Input: part model. Units: mm. Frame: model coordinates. Face numbers are marked on the shaded views. A direction names the side the tool comes from. Coordinates: 2 decimals unless noted, no trailing zeros. Write each loop counter-clockwise with the first axis right and the second up, starting at its lowest first coordinate (ties: lowest second). Pieces come first, ordered by that corner, then holes. Notation, with made-up numbers: (70, 75) - (118, 75) arc R29 ccw to (118, 107) - close; hole circle Ø11 at (-34, 15). An arc over 180 degrees is marked (long way). One line per question, with ' | ' between items. Start each with the question number.
1) First-contact query: P1, Ø3, axis at x = 81, z = -27.5, coming from the -Y side; P2, Ø9.5, axis at x = -136.5, z = -240, coming from the +Y side; P3, Ø15, axis at x = -132.5, z = -236, coming from the -Y side. Flat tips, straight axial feed; report the tip coordinate or a pass-through.
2) Draft query along Z for the marked faces 4, 5, 6 and 7. Return one class per face: released by +Z, released by -Z, zero draft, split by the parting line, or undercut.
3) Line query: line 1 (Y direction, x = 48.5, z = -10); line 2 (X direction, y = -253, z = 18); line 3 (X direction, y = 6.5, z = 45). Output: solid intervals per line, ascending.
4) Section query B-B on x = 0. Return loops of the section in (y, z), and give its area (3 significant figures).
5) Section query A-A on z = 0. Return loops of the section in (x, y).
6) Section query C-C on y = -152.5. Return loops of the section in (x, z).
7) Reachability of the marked faces 1, 2 and 3 from +Z, -Z, +X, -X, +Y, -Y: full face, straight path, thin tool, end or side. Return the list, or none.
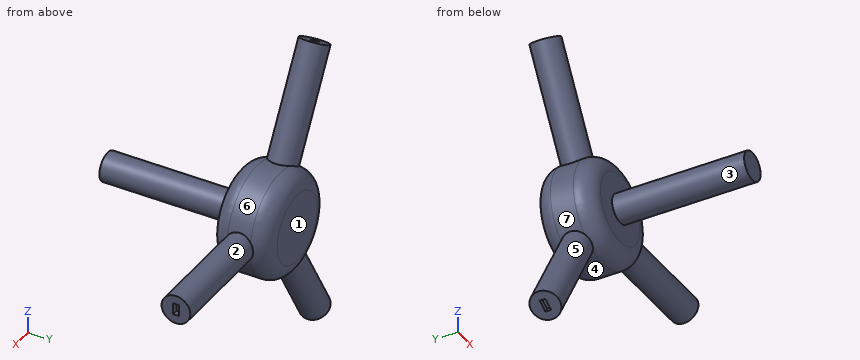
```python
from build123d import *

# Parameters (mm, degrees)
SKETCH_1_W               = 25
SKETCH_1_H               = 230
SKETCH_5_R               = 25
EXTRUDE_1_DEPTH          = 280
PATTERN_CIRCULAR_1_COUNT = 3
SKETCH_7_W               = 20
SKETCH_7_H               = 10
CUT_EXTRUDE_2_DEPTH      = 10
PATTERN_CIRCULAR_2_COUNT = 3


with BuildPart() as part:
    # 草图1 → 旋转1 (revolve)
    with BuildSketch(Plane.XY, mode=Mode.PRIVATE) as revolve_1_sk:
        with BuildLine():
            Line((90, -20), (90, 20))
            ThreePointArc((90, 20), (81.213203436, 41.213203436), (60, 50))
            Line((60, 50), (0, 50))
            Line((0, 50), (0, -50))
            Line((0, -50), (60, -50))
            ThreePointArc((60, -50), (81.213203436, -41.213203436), (90, -20))
        make_face()
        with Locations((12.5, -165)):
            Rectangle(SKETCH_1_W, SKETCH_1_H)
    revolve(revolve_1_sk.sketch.rotate(Axis((0, 124, 0), (0, -1, 0)), 90), axis=Axis((0, 124, 0), (0, -1, 0)))

    # 草图5 → 凸台-拉伸1 (add)
    with BuildSketch(Plane(origin=(0, 0, 0), x_dir=(0, 0, -1), z_dir=(1, 0, 0))):
        with Locations(Location((0, 0, 0), (0, 0, 126.869897646))):
            Circle(SKETCH_5_R)
    extrude_1 = extrude(amount=EXTRUDE_1_DEPTH)

    # 阵列(圆周)1: 凸台-拉伸1 ×3 about axis
    pattern_circular_1_axis = Axis((0, 0, 0), (0, 1, 0))
    for i in range(1, PATTERN_CIRCULAR_1_COUNT):
        add(extrude_1.rotate(pattern_circular_1_axis, i * 360 / PATTERN_CIRCULAR_1_COUNT))

    # 草图7 → 切除-拉伸2 (cut)
    with BuildSketch(Plane(origin=(280, 0, 0), x_dir=(0, 0, -1), z_dir=(1, 0, 0))):
        Rectangle(SKETCH_7_W, SKETCH_7_H)
    cut_extrude_2 = extrude(amount=-CUT_EXTRUDE_2_DEPTH, mode=Mode.SUBTRACT)

    # 阵列(圆周)2: 切除-拉伸2 ×3 about axis
    pattern_circular_2_axis = Axis((0, 0, 0), (0, 1, 0))
    for i in range(1, PATTERN_CIRCULAR_2_COUNT):
        add(cut_extrude_2.rotate(pattern_circular_2_axis, i * 360 / PATTERN_CIRCULAR_2_COUNT), mode=Mode.SUBTRACT)


solid = part.part
```
Answer key:
1) P1: y = -37.95 | P2: y = 25 | P3: y = -25
2) face 4: released by -Z | face 5: undercut | face 6: released by +Z | face 7: undercut
3) line 1: -50 to 50 | line 2: -17.35 to 17.35 | line 3: -77.94 to 77.94
4) outline: (-280, -25) - (-50, -25) - (-50, -60) arc R30 ccw to (-20, -90) - (20, -90) arc R30 ccw to (50, -60) - (50, 60) arc R30 ccw to (20, 90) - (-20, 90) arc R30 ccw to (-50, 60) - (-50, 25) - (-280, 25) - close | area: 28,700 mm²
5) outline: (-90, -20) arc R30 ccw to (-60, -50) - (-25, -50) - (-25, -280) - (25, -280) - (25, -50) - (60, -50) arc R30 ccw to (89.58, -25) - (280, -25) - (280, -5) - (270, -5) - (270, 5) - (280, 5) - (280, 25) - (89.58, 25) arc R30 ccw to (60, 50) - (-60, 50) arc R30 ccw to (-90, 20) - close
6) outline: circle Ø50 at (0, 0)
7) face 1: +Z, -Z, +X, -X, +Y | face 2: +X | face 3: -Y
